Study the drawing (mm; zero at the part's minimum x, y, z) and answer. Coordinates: 2 decimals unless noted, no trailing zeros. Write each loop counter-clockwise with the first axis right and the second up, starting at its lowest first coordinate (ties: lowest second). Pieces come first, ordered by that corner, then holes. Notation, with made-up numbers: M 56.25,-29.5 L 76.25,-29.5 A28 ccw 76.25,9.5 Z; hole C -31.5,-2.75 d6. An arc over 180 degrees is marked long. Answer as CSV lines item,"result". Start each with the question number.
(1) Flat-ended cylindrical pins translate along their axes: P1, Ø1.5, axis at x = 91, y = 187, coming from the -Z side; P2, Ø3, axis at y = 173, z = 4, coming from the -X side (1 decimal); P3, Ø4, axis at y = 78.5, z = 7, coming from the -X side (1 decimal); P4, Ø5, axis at x = 157, z = 7, coming from the -Y side. Find the tip coordinate at first contact, or state that the pin passes through.
(2) A cutting plane is placed at B-B on y = 111. Give the vertices of the cut face in (x, z) (1 decimal).
(3) A cutting plane is placed at A-A on z = 4.75. Give the vertices of the cut face in (x, y) (1 decimal).
(4) Find the intervals of material crossed by L1, parallel to Y at x = 366.5, z = 15; L2, parallel to Y at x = 260.5, z = 8 (1 decimal); L3, parallel to X at y = 254, z = 5.5 (1 decimal), in increasing order. Write a range as [from, to].
(5) A cutting plane is placed at C-C on x = 101.5. Give the vertices of the cut face in (y, z) (1 decimal).
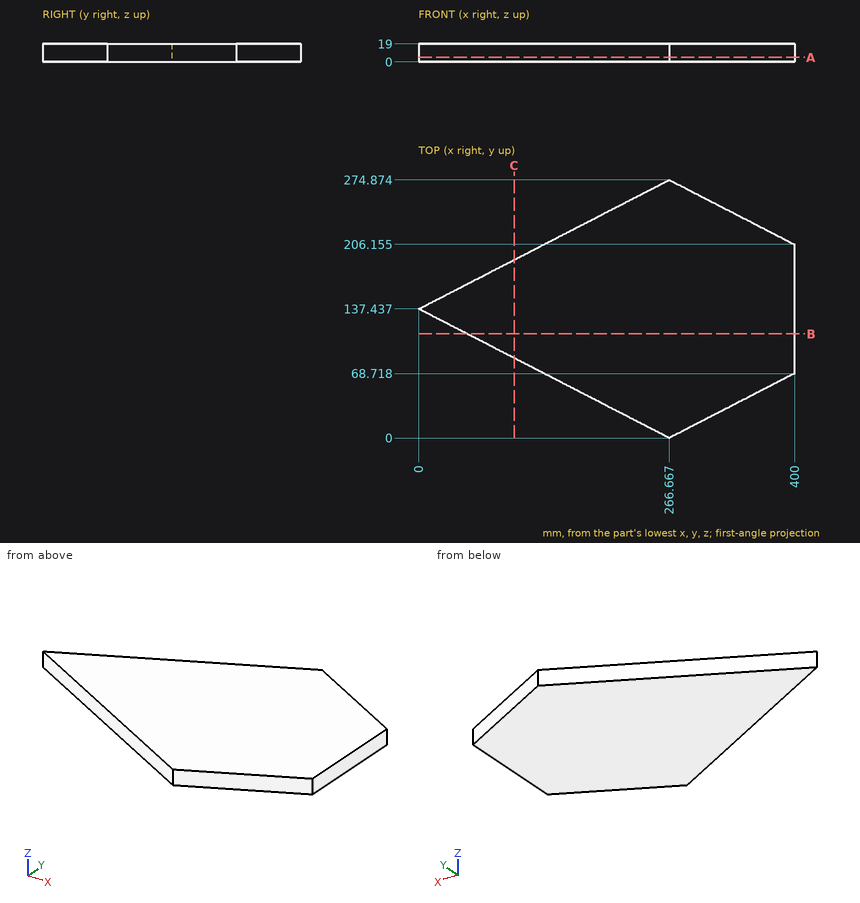
Here are the results:
1,P1,"passes through"
1,P2,"stops at x = 66.1"
1,P3,"stops at x = 110.5"
1,P4,"stops at y = 55.23"
2,outline,"M 51.3,0 L 400,0 L 400,19 L 51.3,19 Z"
3,outline,"M 0,137.4 L 266.7,0 L 400,68.7 L 400,206.2 L 266.7,274.9 Z"
4,L1,"y = [51.45, 223.42]"
4,L2,"y = [3.2, 271.7]"
4,L3,"x = [226.2, 307.2]"
5,outline,"M 85.1,0 L 189.7,0 L 189.7,19 L 85.1,19 Z"
